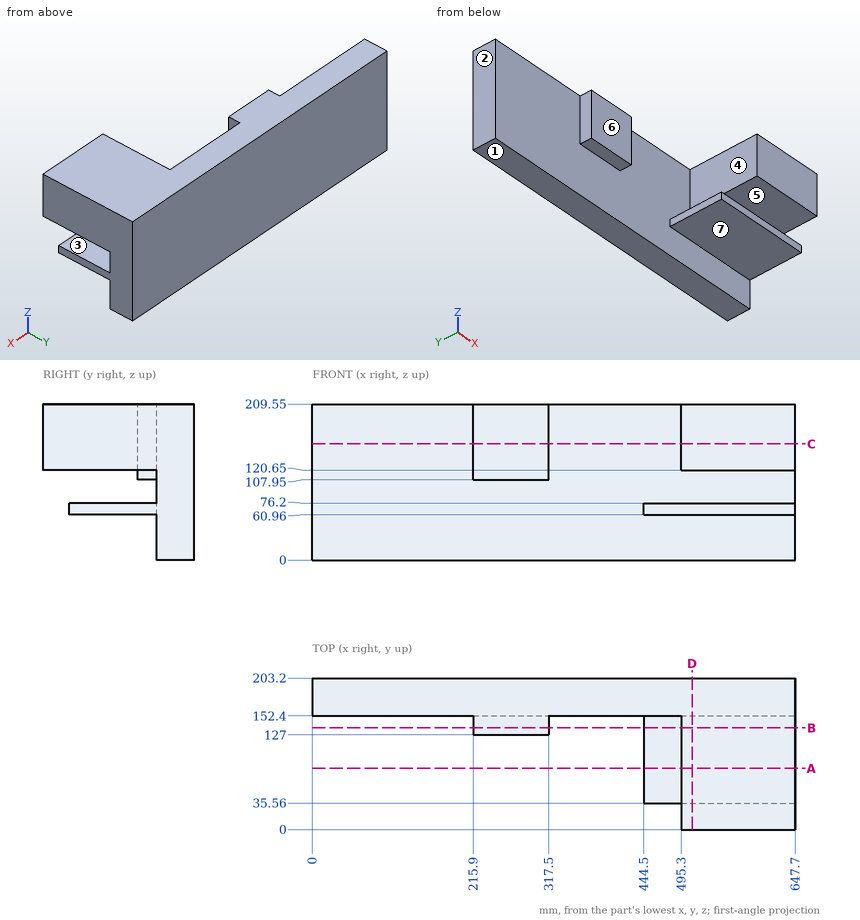
Study the drawing (mm; zero at the part's minimum x, y, z) and answer. A direction names the side the tool comes from. Round coordinates to 2 decimals unless told otherwise and drop trailing zeros. Write each loop counter-clockwise with the first axis right and the second up, starting at its lowest first coordinate (ties: lowest second). Pieces come first, ordered by that corner, then holes. Notation, with made-up numbers: (86.5, 21.5) - (134.5, 21.5) arc R19 ccw to (134.5, 40.5) - close; hole circle Ø8 at (85.25, -8). An arc over 180 degrees is marked (long way). Use a Markdown table: item, result. Add a question column.
1. For a pull along Z with two mould halves and no side action, classify the marked faces 1, 2 and 3 as +Z half, -Z half, draft (parallel to the pull), parting line (faces both ways), or undercut.
2. A tool of negligible diameter and unlimited length cuts with its end or side. For the marked faces 4, 5, 6 and 7, from which of +Z, -Z, +X, -X, +Y, -Y can it reach the whole face along a straight path? Write none if from no direction.
3. The part is cut by section A-A (y = 82). Write down the section's boundary in (x, z), and give its area (3 significant figures).
4. The part is cut by section C-C (z = 156). Write down the section's boundary in (x, y), and give its area (3 significant figures).
5. Consider line 1 (Z direction, x = 511.5, y = 97); line 2 (X direction, y = 150.5, z = 199); line 3 (Y direction, x = 503.5, z = 97). Determine where each line is inside the solid, lowest interval first.
6. The part is cut by section B-B (y = 136.5). Write down the section's boundary in (x, z).
7. The part is cut by section D-D (x = 509.5). Write down the section's boundary in (y, z), and give its area (3 significant figures).
8. Flat-ended cylindrical pins translate along their axes: P1, Ø12.5, axis at x = 249.5, y = 136, coming from the -Z side; P2, Ø4.5, axis at x = 593.5, z = 66, coming from the -Y side; P3, Ø10, axis at y = 101, z = 55, coming from the -X side; P4, Ø12, axis at y = 117, z = 72, coming from the -X side. Find the tip coordinate at first contact, or state that the pin passes through.
Reported:
| question | item | result |
|---|---|---|
| 1 | face 1 | -Z half |
| 1 | face 2 | draft |
| 1 | face 3 | undercut |
| 2 | face 4 | +Z, -Y |
| 2 | face 5 | +X, -Y |
| 2 | face 6 | +Z, -Z, -X, -Y |
| 2 | face 7 | -Z, +X, -X, -Y |
| 3 | outline | (444.5, 60.96) - (647.7, 60.96) - (647.7, 76.2) - (444.5, 76.2) - close; (495.3, 120.65) - (647.7, 120.65) - (647.7, 209.55) - (495.3, 209.55) - close |
| 3 | area | 16,600 mm^2 |
| 4 | outline | (0, 152.4) - (215.9, 152.4) - (215.9, 127) - (317.5, 127) - (317.5, 152.4) - (495.3, 152.4) - (495.3, 0) - (647.7, 0) - (647.7, 203.2) - (0, 203.2) - close |
| 4 | area | 58,700 mm^2 |
| 5 | line 1 | 60.96 to 76.2, 120.65 to 209.55 |
| 5 | line 2 | 215.9 to 317.5, 495.3 to 647.7 |
| 5 | line 3 | 152.4 to 203.2 |
| 6 | outline | (215.9, 107.95) - (317.5, 107.95) - (317.5, 209.55) - (215.9, 209.55) - close; (444.5, 60.96) - (647.7, 60.96) - (647.7, 76.2) - (444.5, 76.2) - close; (495.3, 120.65) - (647.7, 120.65) - (647.7, 209.55) - (495.3, 209.55) - close |
| 7 | outline | (0, 120.65) - (152.4, 120.65) - (152.4, 76.2) - (35.56, 76.2) - (35.56, 60.96) - (152.4, 60.96) - (152.4, 0) - (203.2, 0) - (203.2, 209.55) - (0, 209.55) - close |
| 7 | area | 26,000 mm^2 |
| 8 | P1 | z = 107.95 |
| 8 | P2 | y = 35.56 |
| 8 | P3 | through |
| 8 | P4 | x = 444.5 |
